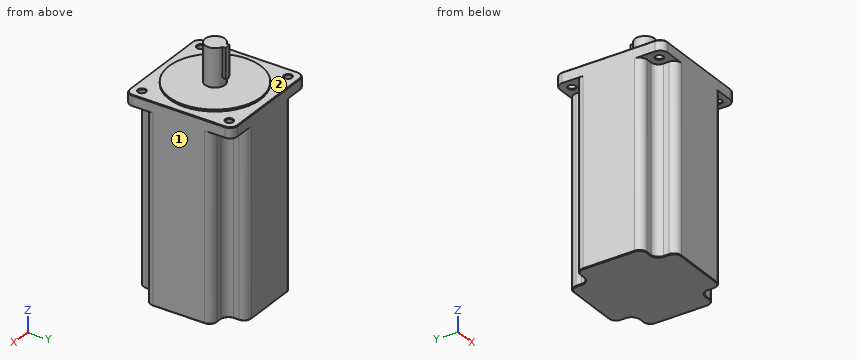
from build123d import *

# Parameters (mm, degrees)
SKETCH1_W                 = 85.85
SKETCH1_H                 = 85.85
BOSS_EXTRUDE1_DEPTH       = 8.38
BOSS_EXTRUDE3_DEPTH       = 147.62
FILLET4_R                 = 6
FILLET5_R                 = 6
SKETCH4_R                 = 36.51
BOSS_EXTRUDE4_DEPTH       = 1.52
SKETCH5_R                 = 7.9375
BOSS_EXTRUDE5_DEPTH       = 30.23
BOSS_EXTRUDE6_DEPTH       = 5
F_5_0MM_DOWEL_HOLE1_D     = 5.5
F_5_0MM_DOWEL_HOLE1_DEPTH = 8.38
CHAMFER1_SIZE             = 0.5


with BuildPart() as part:
    # Sketch1 → Boss-Extrude1 (new body)
    with BuildSketch(Plane.XY):
        Rectangle(SKETCH1_W, SKETCH1_H)
    extrude(amount=-BOSS_EXTRUDE1_DEPTH)

    # Sketch2 → Boss-Extrude3 (add)
    with BuildSketch(Plane(origin=(0, 0, -8.38), x_dir=(-1, 0, 0), z_dir=(0, 0, -1))):
        Polygon((-26.575, -42.925), (26.575, -42.925), (26.575, -26.575), (42.925, -26.575), (42.925, 26.575), (26.575, 26.575), (26.575, 42.925), (-26.575, 42.925), (-26.575, 26.575), (-42.925, 26.575), (-42.925, -26.575), (-26.575, -26.575), align=None)
    extrude(amount=BOSS_EXTRUDE3_DEPTH)

    # Fillet4
    fillet4_edges = [part.edges().sort_by_distance(p)[0] for p in [
        (42.925, -26.575, -82.19),
        (26.575, -26.575, -82.19),
        (26.575, -42.925, -82.19),
        (-26.575, -42.925, -82.19),
        (-26.575, -26.575, -82.19),
        (-42.925, -26.575, -82.19),
        (-42.925, 26.575, -82.19),
        (-26.575, 26.575, -82.19),
        (-26.575, 42.925, -82.19),
        (26.575, 42.925, -82.19),
        (26.575, 26.575, -82.19),
        (42.925, 26.575, -82.19),
    ]]
    fillet(fillet4_edges, radius=FILLET4_R)

    # Fillet5
    fillet5_edges = [part.edges().sort_by_distance(p)[0] for p in [
        (-42.925, -42.925, -4.19),
        (42.925, -42.925, -4.19),
        (42.925, 42.925, -4.19),
        (-42.925, 42.925, -4.19),
    ]]
    fillet(fillet5_edges, radius=FILLET5_R)

    # Sketch4 → Boss-Extrude4 (add)
    with BuildSketch(Plane.XY):
        Circle(SKETCH4_R)
    extrude(amount=BOSS_EXTRUDE4_DEPTH)

    # Sketch5 → Boss-Extrude5 (add)
    with BuildSketch(Plane.XY.offset(1.52)):
        Circle(SKETCH5_R)
    extrude(amount=BOSS_EXTRUDE5_DEPTH)

    # Sketch6 → Boss-Extrude6 (add)
    with BuildSketch(Plane(origin=(0, 9.9375, 0), x_dir=(1, 0, 0), z_dir=(0, 1, 0))):
        with BuildLine():
            Line((-2.5, -31.75), (2.5, -31.75))
            Line((2.5, -31.75), (2.5, -9.25))
            ThreePointArc((2.5, -9.25), (0, -6.75), (-2.5, -9.25))
            Line((-2.5, -9.25), (-2.5, -31.75))
        make_face()
    extrude(amount=-BOSS_EXTRUDE6_DEPTH)

    # Ø5.0mm Dowel Hole1
    with Locations(Plane.XY):
        with Locations((-34.75, 34.75), (34.75, 34.75), (34.75, -34.75), (-34.75, -34.75)):
            Hole(F_5_0MM_DOWEL_HOLE1_D / 2, depth=F_5_0MM_DOWEL_HOLE1_DEPTH)

    # Chamfer1
    chamfer1_edges = [part.edges().sort_by_distance(p)[0] for p in [
        (-42.925, 0, 0),
        (42.925, 0, 0),
        (0, 42.925, 0),
        (0, -42.925, 0),
        (-41.167640687, 41.167640687, 0),
        (41.167640687, 41.167640687, 0),
        (41.167640687, -41.167640687, 0),
        (-41.167640687, -41.167640687, 0),
        (-32, -34.75, 0),
        (-32, -34.75, -8.38),
        (37.5, -34.75, 0),
        (37.5, -34.75, -8.38),
        (37.5, 34.75, 0),
        (37.5, 34.75, -8.38),
        (-32, 34.75, 0),
        (-32, 34.75, -8.38),
        (34.75, -26.575, -156),
        (42.925, 0, -156),
        (26.575, 34.75, -156),
        (34.75, 26.575, -156),
        (26.575, -34.75, -156),
        (0, -42.925, -156),
        (-26.575, -34.75, -156),
        (-34.75, -26.575, -156),
        (-42.925, 0, -156),
        (-34.75, 26.575, -156),
        (-26.575, 34.75, -156),
        (0, 42.925, -156),
        (41.167640687, 24.817640687, -156),
        (24.817640687, 41.167640687, -156),
        (-24.817640687, 41.167640687, -156),
        (-41.167640687, 24.817640687, -156),
        (-41.167640687, -24.817640687, -156),
        (-24.817640687, -41.167640687, -156),
        (24.817640687, -41.167640687, -156),
        (41.167640687, -24.817640687, -156),
        (28.332359313, -28.332359313, -156),
        (-28.332359313, -28.332359313, -156),
        (-28.332359313, 28.332359313, -156),
        (28.332359313, 28.332359313, -156),
    ]]
    chamfer(chamfer1_edges, length=CHAMFER1_SIZE)


solid = part.part
Input: part model. Units: mm. Frame: model coordinates. Face numbers are marked on the shaded views. A direction names the side the tool comes from. Give positions to 0.01 mm unless a question says otherwise; leave off trailing zeros. Order: outer loops, then holes, each group sorted by start corner. A loop starts at its lowest first (then second) coordinate and runs counter-clockwise, first axis right, second up.
Q1. Section B-B on z = -51.5. Output: boundary loops of the cut face in (x, y) (3 decimals), and give its area (3 significant figures).
Checked values:
outline: (-42.925, -20.575) arc R6 ccw to (-36.925, -26.575) - (-32.575, -26.575) arc R6 cw to (-26.575, -32.575) - (-26.575, -36.925) arc R6 ccw to (-20.575, -42.925) - (20.575, -42.925) arc R6 ccw to (26.575, -36.925) - (26.575, -32.575) arc R6 cw to (32.575, -26.575) - (36.925, -26.575) arc R6 ccw to (42.925, -20.575) - (42.925, 20.575) arc R6 ccw to (36.925, 26.575) - (32.575, 26.575) arc R6 cw to (26.575, 32.575) - (26.575, 36.925) arc R6 ccw to (20.575, 42.925) - (-20.575, 42.925) arc R6 ccw to (-26.575, 36.925) - (-26.575, 32.575) arc R6 cw to (-32.575, 26.575) - (-36.925, 26.575) arc R6 ccw to (-42.925, 20.575) - close
area: 6,270 mm2
Q2. Contact query for flat-ended pins moving along their axis: pin 1 Ø2 at (y, z) = (-35, -112) entering from -X (3 decimals); pin 2 Ø5.5 at (x, z) = (-0.5, 25.5) entering from +Y; pin 3 Ø7 at (x, y) = (34.75, 34.75) entering from +Z. Output: stop coordinate, or through.
Checked values:
pin 1: stops at x = -26.575
pin 2: stops at y = 9.94
pin 3: stops at z = 0
Q3. Section D-D on x = -12.5. Output: boundary loops of the cut face in (y, z) (1 decimal), and give its area (3 significant figures).
Checked values:
outline: (-42.9, -155.5) - (-42.4, -156) - (42.4, -156) - (42.9, -155.5) - (42.9, -0.5) - (42.4, 0) - (34.3, 0) - (34.3, 1.5) - (-34.3, 1.5) - (-34.3, 0) - (-42.4, 0) - (-42.9, -0.5) - close
area: 13,500 mm2
Q4. Set-up query: the marked faces 1 and 2. Return all of +Z, -Z, +X, -X, +Y, -Y with unobstructed straight access to the full face (end or side cutting, diameter ignored); none if empty.
Checked values:
face 1: +Z, -Z, +X, +Y, -Y
face 2: +Z
Q5. Ray query, probe 1 along Y at (x, z) = (-34.75, -2.5) (3 decimals); probe 2 along X at (y, z) = (32, -62.5); probe 3 along Z at (x, y) = (12.5, 39). Return the intervals inside material, ascending.
Checked values:
probe 1: y = -42.925 to -37.5, -32 to 32, 37.5 to 42.925
probe 2: x = -26.6 to 26.6
probe 3: z = -156 to 0
